Input: part model. Units: mm. Frame: model coordinates. Face numbers are marked on the shaded views. A direction names the side the tool comes from. Give positions to 0.01 mm unless a question says otherwise; leave off trailing zeros. Order: outer loops, then holes, each group sorted by start corner. A loop starts at its lowest first (then second) coordinate and runs counter-clockwise, first axis right, second up. Notation, with made-up numbers: M 26.5,70.5 L 83.5,70.5 A21 cw 83.5,86.5 Z; hole C 77,81 d3. An arc over 180 degrees is marked long. Use a Markdown table: item, result.
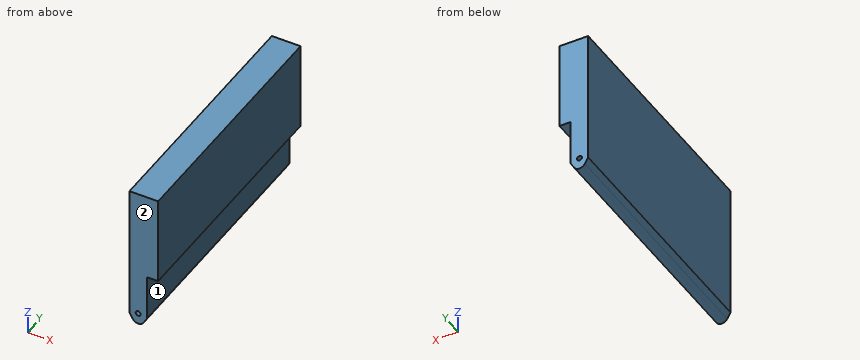
from build123d import *

# Parameters (mm, degrees)
SKETCH1_W           = 22
SKETCH1_H           = 120
BOSS_EXTRUDE1_DEPTH = 200
SKETCH2_OUTSIDE_W   = 70.854
SKETCH2_OUTSIDE_H   = 168.854
CUT_EXTRUDE1_DEPTH  = 210.095671883
FILLET1_R           = 5
CUT_EXTRUDE2_DEPTH  = 210.095671883
SKETCH4_W           = 96.947441117
SKETCH4_H           = 200
BOSS_EXTRUDE2_DEPTH = 5
SKETCH5_W           = 4
SKETCH5_H           = 96.947441117
CUT_EXTRUDE3_DEPTH  = 210.418241803
SKETCH6_R           = 2
CUT_EXTRUDE4_DEPTH  = 210.418241803
SKETCH8_W           = 9
SKETCH8_H           = 26
CUT_EXTRUDE5_DEPTH  = 210.418241803


with BuildPart() as part:
    # Sketch1 → Boss-Extrude1 (new body)
    with BuildSketch(Plane(origin=(0, 0, 0), x_dir=(1, 0, 0), z_dir=(0, 1, 0))):
        Rectangle(SKETCH1_W, SKETCH1_H)
    extrude(amount=BOSS_EXTRUDE1_DEPTH)

    # Sketch2 outside → Cut-Extrude1 (cut, through all)
    with BuildSketch(Plane(origin=(0, 200, 0), x_dir=(1, 0, 0), z_dir=(0, 1, 0))):
        Rectangle(SKETCH2_OUTSIDE_W, SKETCH2_OUTSIDE_H)
        Polygon((0, 60), (-11, 40.947441117), (-11, -60), (11, -60), (11, 40.947441117), align=None, mode=Mode.SUBTRACT)
    extrude(amount=-CUT_EXTRUDE1_DEPTH, mode=Mode.SUBTRACT)

    # Fillet1
    fillet1_edges = [part.edges().sort_by_distance(p)[0] for p in [
        (0, 100, -60),
    ]]
    fillet(fillet1_edges, radius=FILLET1_R)

    # Sketch3 → Cut-Extrude2 (cut, through all)
    with BuildSketch(Plane(origin=(0, 200, 0), x_dir=(1, 0, 0), z_dir=(0, 1, 0))):
        Polygon((-11, 36.947441117), (-7, 36.947441117), (-7, 47.875644347), (-11, 40.947441117), align=None)
        Polygon((7, 47.875644347), (11, 40.947441117), (11, 36.947441117), (7, 36.947441117), align=None)
    extrude(amount=-CUT_EXTRUDE2_DEPTH, mode=Mode.SUBTRACT)

    # Sketch4 → Boss-Extrude2 (add)
    with BuildSketch(Plane(origin=(11, 0, 0), x_dir=(0, 0, -1), z_dir=(1, 0, 0))):
        with Locations((-11.526279442, 100)):
            Rectangle(SKETCH4_W, SKETCH4_H)
    extrude(amount=BOSS_EXTRUDE2_DEPTH)

    # Sketch5 → Cut-Extrude3 (cut, through all)
    with BuildSketch(Plane(origin=(0, 200, 0), x_dir=(1, 0, 0), z_dir=(0, 1, 0))):
        with Locations((-9, -11.526279442)):
            Rectangle(SKETCH5_W, SKETCH5_H)
    extrude(amount=-CUT_EXTRUDE3_DEPTH, mode=Mode.SUBTRACT)

    # Sketch6 → Cut-Extrude4 (cut, through all)
    with BuildSketch(Plane(origin=(0, 200, 0), x_dir=(1, 0, 0), z_dir=(0, 1, 0))):
        with Locations(Location((0, 46, 0), (0, 0, 270))):
            Circle(SKETCH6_R)
    extrude(amount=-CUT_EXTRUDE4_DEPTH, mode=Mode.SUBTRACT)

    # Sketch8 → Cut-Extrude5 (cut, through all)
    with BuildSketch(Plane(origin=(0, 200, 0), x_dir=(1, 0, 0), z_dir=(0, 1, 0))):
        with Locations((11.5, 23.947441117)):
            Rectangle(SKETCH8_W, SKETCH8_H)
    extrude(amount=-CUT_EXTRUDE5_DEPTH, mode=Mode.SUBTRACT)


solid = part.part
1) Reachability of the marked faces 1 and 2 from +Z, -Z, +X, -X, +Y, -Y: full face, straight path, thin tool, end or side. Return the list, or none.
Response values:
| item | result |
|---|---|
| face 1 | -Z, +X, +Y, -Y |
| face 2 | +Z, -Z, +X, -X, -Y |
2) Material intervals for line 1 (X direction, y = 112, z = -46); line 2 (X direction, y = 41.5, z = -18); line 3 (Z direction, x = 10.5, y = 36), sorted ascending. Write a range as from..to.
Response values:
| item | result |
|---|---|
| line 1 | x = -7..-2, 2..7 |
| line 2 | x = -7..7 |
| line 3 | z = -10.95..60 |
3) Cut plane A-A on z = -46. Return loops of the section in (x, y), and give its area (3 significant figures).
Response values:
| item | result |
|---|---|
| outline | M -7,0 L -2,0 L -2,200 L -7,200 Z; M 2,0 L 7,0 L 7,200 L 2,200 Z |
| area | 2,000 mm² |
4) Cut plane D-D on z = -17.5. Return loops of the section in (x, y), and give its area (3 significant figures).
Response values:
| item | result |
|---|---|
| outline | M -7,0 L 7,0 L 7,200 L -7,200 Z |
| area | 2,800 mm² |
5) First-contact query: pin 1 Ø2.5 at (x, y) = (13.5, 114.5) entering from -Z; pin 2 Ø18.5 at (y, z) = (66, -33.5) entering from +X. Flat tips, straight axial feed; report the tip coordinate or a pass-through.
Response values:
| item | result |
|---|---|
| pin 1 | stops at z = -10.95 |
| pin 2 | stops at x = 7 |
6) Cut plane B-B on x = 0. Return loops of the section in (y, z), and give its area (3 significant figures).
Response values:
| item | result |
|---|---|
| outline | M 0,-55 L 200,-55 L 200,-48 L 0,-48 Z; M 0,-44 L 200,-44 L 200,60 L 0,60 Z |
| area | 22,200 mm² |
7) Cut plane C-C on y = 59.5. Return loops of the section in (x, z).
Response values:
| item | result |
|---|---|
| outline | M -7,-47.88 L -4.33,-52.5 A5 ccw 4.33,-52.5 L 7,-47.88 L 7,-10.95 L 16,-10.95 L 16,60 L -7,60 Z; hole C 0,-46 d4 |
